Autodesk Inventor part; units mm, degrees
ref_plane "YZ Plane" through (0, 0, 0) normal (1, 0, 0) x (0, 1, 0)
ref_plane "XZ Plane" through (0, 0, 0) normal (0, 1, 0) x (-1, 0, 0)
ref_plane "XY Plane" through (0, 0, 0) normal (0, 0, 1) x (1, 0, 0)
sketch "草图1" plane through (0, 0, 0) normal (0, 0, 1) x (1, 0, 0)
  line L0 (-50, -50) -> (50, -50)
  line L1 (50, -50) -> (50, 50)
  line L2 (50, 50) -> (-50, 50)
  line L3 (-50, 50) -> (-50, -50)
  line L4 (-50, -50) -> (50, 50) construction
  line L5 (50, -50) -> (-50, 50) construction
  line L6 (-50, -50) -> (50, -50)
  line L7 (50, -50) -> (50, -65)
  line L8 (50, -65) -> (-50, -65)
  line L9 (-50, -65) -> (-50, -50)
  point P0 (0, 0)
  dimension "d0" = 100
  dimension "d1" = 100
  dimension "d2" = 15
extrude "拉伸1" add sketch "草图1" along normal blind 6
sketch "草图2" plane through (0, 0, 6) normal (0, 0, 1) x (1, 0, 0)
  line L0 (-25, -25) -> (25, -25)
  line L1 (25, -25) -> (25, 25)
  line L2 (25, 25) -> (-25, 25)
  line L3 (-25, 25) -> (-25, -25)
  line L4 (-25, -25) -> (25, 25) construction
  line L5 (25, -25) -> (-25, 25) construction
  point P0 (0, 0)
  dimension "d5" = 50
  dimension "d6" = 50
extrude "拉伸2" add sketch "草图2" along normal blind 6
sketch "草图3" plane through (0, 0, 12) normal (0, 0, 1) x (1, 0, 0)
  line L0 (-17.5, -17.5) -> (17.5, -17.5)
  line L1 (17.5, -17.5) -> (17.5, 17.5)
  line L2 (17.5, 17.5) -> (-17.5, 17.5)
  line L3 (-17.5, 17.5) -> (-17.5, -17.5)
  line L4 (-17.5, -17.5) -> (17.5, 17.5) construction
  line L5 (17.5, -17.5) -> (-17.5, 17.5) construction
  point P0 (0, 0)
  dimension "d9" = 35
  dimension "d10" = 35
extrude "拉伸3" cut sketch "草图3" against normal through all
sketch "草图4" plane through (0, 0, 12) normal (0, 0, 1) x (1, 0, 0)
  line L0 (-21, -21) -> (21, -21)
  line L1 (21, -21) -> (21, 21)
  line L2 (21, 21) -> (-21, 21)
  line L3 (-21, 21) -> (-21, -21)
  line L4 (-21, -21) -> (21, 21) construction
  line L5 (21, -21) -> (-21, 21) construction
  circle A0 centre (21, 21) radius 2.15
  circle A1 centre (-21, 21) radius 2.15
  circle A2 centre (-21, -21) radius 2.15
  circle A3 centre (21, -21) radius 2.15
  point P0 (0, 0)
  dimension "d13" = 42
  dimension "d14" = 42
  dimension "d15" = 4.3
  dimension "d16" = 4.3
  dimension "d17" = 4.3
  dimension "d18" = 4.3
extrude "拉伸4" cut sketch "草图4" against normal through all contours L3 A2 L0 | L0 A2 L3 | A3 L1 L0 | L0 L1 A3 | A1 L2 L3 | L3 L2 A1 | A0 L2 L1 | L1 L2 A0
sketch "草图5" plane through (0, 0, 0) normal (0, 0, -1) x (-1, 0, 0)
  line L0 (0, 0) -> (15, 0)
  line L1 (15, -17.5) -> (15, -57.5)
  line L2 (15, -57.5) -> (0, -57.5)
  line L3 (-17.5, -17.5) -> (17.5, -17.5)
  line L4 (15, -17.5) -> (0, -17.5)
  line L5 (-15, -17.5) -> (-15, -57.5)
  line L6 (-15, -57.5) -> (0, -57.5)
  line L7 (17.5, -17.5) -> (-17.5, -17.5)
  line L8 (0, -57.5) -> (10, -57.5)
  line L9 (10, -57.5) -> (10, -76.7389)
  line L10 (10, -76.7389) -> (0, -76.7389)
  line L11 (0, -76.7389) -> (0, -57.5)
  line L12 (-10, -57.5) -> (-10, -76.7389)
  line L13 (-10, -76.7389) -> (0, -76.7389)
  dimension "d21" = 15
  dimension "d22" = 40
  dimension "d23" = 10
extrude "拉伸5" cut sketch "草图5" against normal blind 3
sketch "草图6" plane through (0, 0, 0) normal (0, 0, -1) x (-1, 0, 0)
  point P0 (0, 0)
sketch "草图7" plane through (-50, -65, 6) normal (0, -1, 0) x (1, 0, 0)
  line L0 (100, -6) -> (0, -6)
  line L1 (0, -6) -> (0, 0)
  line L2 (100, -6) -> (0, -6)
  line L3 (0, -6) -> (0, 0)
  line L4 (0, 0) -> (100, 0)
  line L5 (100, 0) -> (100, -6)
  point P0 (50, -6)
extrude "拉伸6" add sketch "草图7" along normal blind 80
sketch "草图8" plane through (0, 0, 0) normal (0, 0, -1) x (-1, 0, 0)
  line L0 (10, -65) -> (-10, -65)
  line L1 (50, 50) -> (50, -145)
  line L2 (0, -65) -> (50, -65)
  line L3 (50, -65) -> (50, -145)
  line L4 (50, -145) -> (0, -145)
  line L5 (0, -145) -> (0, -65)
  line L6 (-50, 50) -> (-50, -145)
  line L7 (0, -65) -> (-50, -65)
  line L8 (-50, -145) -> (0, -145)
  point P0 (0, 0)
extrude "拉伸7" cut sketch "草图8" against normal blind 3
sketch "草图9" plane through (0, 0, 3) normal (0, 0, -1) x (-1, 0, 0)
  line L0 (-50, -145) -> (-50, -65)
  line L1 (-50, -65) -> (-47, -65)
  line L2 (-47, -65) -> (-47, -142)
  line L3 (-47, -155.7604) -> (-50, -155.7604)
  line L4 (-50, -145) -> (-50, -65)
  line L5 (50, 50) -> (50, -145)
  line L6 (50, -65) -> (47, -65)
  line L7 (47, -65) -> (47, -142)
  line L8 (47, -155.7604) -> (50, -155.7604)
  line L9 (50, -145) -> (50, -65)
  line L10 (-47, -142) -> (47, -142)
  line L11 (63.4475, -142) -> (63.4475, -145)
  line L12 (50, -145) -> (-50, -145)
  line L13 (-50, -145) -> (-50, -142)
  point P0 (0, 0)
  point P1 (50, -145)
  dimension "d30" = 3
  dimension "d31" = 3
  dimension "d32" = 3
extrude "拉伸8" add sketch "草图9" along normal blind 50
sketch "草图10" plane through (0, 0, -47) normal (0, 0, -1) x (-1, 0, 0)
  line L0 (50, -65) -> (47, -65)
  line L1 (50, -145) -> (50, -65)
  line L2 (-50, 50) -> (-50, -145)
  line L3 (-50, -145) -> (50, -145)
  line L4 (50, -145) -> (50, -65)
  line L5 (50, -65) -> (-50, -65)
  line L6 (-50, -65) -> (-50, -145)
  point P0 (0, 0)
extrude "拉伸9" add sketch "草图10" along normal blind 3
sketch "草图11" plane through (-50, 50, 0) normal (-1, 0, 0) x (0, 0, 1)
  line L0 (-42.728, -178.1257) -> (-27.728, -178.1257)
  line L1 (-27.728, -178.1257) -> (-27.728, -188.1257)
  line L2 (-27.728, -188.1257) -> (-42.728, -188.1257)
  line L3 (-42.728, -188.1257) -> (-42.728, -178.1257)
  point P0 (0, -50)
  dimension "d37" = 10
  dimension "d38" = 15
extrude "拉伸10" cut sketch "草图11" against normal blind 3
sketch "草图12" plane through (-50, -145, 6) normal (0, -1, 0) x (1, 0, 0)
  line L0 (0, -56) -> (100, -56)
  line L1 (100, -6) -> (100, -56)
  line L2 (100, -6) -> (97, -6)
  line L3 (100, -6) -> (100, -56)
  line L4 (0, -56) -> (100, -56)
  line L5 (0, -6) -> (0, -56)
  line L6 (3, -6) -> (0, -6)
  line L7 (3, -6) -> (3, -53)
  line L8 (3, -53) -> (97, -53)
  line L9 (97, -6) -> (97, -53)
  line L10 (100, -56) -> (0, -56)
  line L11 (0, -56) -> (0, -6)
  line L12 (0, -6) -> (100, -6)
  line L13 (100, -6) -> (100, -56)
  point P0 (50, -6)
sketch "草图13" plane through (0, 0, -50) normal (0, 0, -1) x (-1, 0, 0)
  line L0 (50, -145) -> (50, -65)
  line L1 (50, -65) -> (-50, -65)
  line L2 (-53.2797, -65) -> (-53.2797, -62)
  line L3 (-50, -62) -> (50, -62)
  line L4 (50, -62) -> (50, -65)
  line L5 (-50, 50) -> (-50, -65)
  line L6 (-50, -62) -> (-50, -65)
  line L7 (-50, 50) -> (-50, -65)
  line L8 (-50, 50) -> (-50, -145)
  line L9 (-50, -65) -> (-50, -145)
  line L10 (-50, 50) -> (-50, -65)
  line L11 (-50, 50) -> (-50, -145)
  line L12 (-50, -65) -> (-50, -145)
  point P0 (0, 0)
  dimension "d41" = 3
sketch "草图14" plane through (0, 0, 0) normal (0, 0, -1) x (-1, 0, 0)
  point P0 (0, 0)
extrude "拉伸11" add sketch "草图13" against normal blind 50
sketch "草图15" plane through (-50, -62, -50) normal (0, 1, 0) x (1, 0, 0)
  line L0 (50, -50) -> (35, -50)
  line L1 (35, -50) -> (35, -38)
  line L2 (35, -38) -> (50, -38)
  line L3 (50, -38) -> (50, -50)
  line L4 (50, -50) -> (65, -50)
  line L5 (65, -50) -> (65, -38)
  line L6 (65, -38) -> (50, -38)
  dimension "d44" = 15
  dimension "d45" = 12
extrude "拉伸12" cut sketch "草图15" against normal blind 10
sketch "草图16" plane through (-50, -145, 6) normal (0, -1, 0) x (1, 0, 0)
  line L0 (50, -6) -> (50, -31)
  line L1 (100, -56) -> (0, -56)
  circle A0 centre (50, -31) radius 3.15
  dimension "d48" = 25
  dimension "d49" = 6.3
extrude "拉伸13" cut sketch "草图16" against normal blind 10
sketch "草图17" plane through (0, 0, 12) normal (0, 0, 1) x (1, 0, 0)
  line L0 (17.5, 17.5) -> (-17.5, 17.5)
  line L1 (-17.5, -17.5) -> (17.5, -17.5)
  line L2 (17.5, -17.5) -> (17.5, 17.5)
  line L3 (17.5, 17.5) -> (-17.5, 17.5)
  line L4 (-17.5, 17.5) -> (-17.5, -17.5)
  line L5 (-17.5, -17.5) -> (17.5, 17.5) construction
  line L6 (17.5, -17.5) -> (-17.5, 17.5) construction
  line L7 (-12.5, -12.5) -> (12.5, -12.5)
  line L8 (12.5, -12.5) -> (12.5, 12.5)
  line L9 (12.5, 12.5) -> (-12.5, 12.5)
  line L10 (-12.5, 12.5) -> (-12.5, -12.5)
  line L11 (-12.5, -12.5) -> (12.5, 12.5) construction
  line L12 (12.5, -12.5) -> (-12.5, 12.5) construction
  point P0 (0, 0)
  dimension "d52" = 25
  dimension "d53" = 25
extrude "拉伸14" add sketch "草图17" against normal blind 12
sketch "草图18" plane through (0, 0, 0) normal (0, 0, -1) x (-1, 0, 0)
  line L0 (-15, -17.5) -> (15, -17.5)
  line L1 (-15, -17.5) -> (15, -17.5)
  line L2 (15, -17.5) -> (15, -12.5)
  line L3 (15, -12.5) -> (-15, -12.5)
  line L4 (-15, -12.5) -> (-15, -17.5)
  point P0 (0, 0)
  point P1 (15, -17.5)
  dimension "d56" = 5
extrude "拉伸15" cut sketch "草图18" against normal blind 3
sketch "草图19" plane through (-50, -62, -50) normal (0, 1, 0) x (1, 0, 0)
  line L0 (35, -50) -> (35, -38)
  line L1 (35, -38) -> (65, -38)
  line L2 (65, -38) -> (65, -50)
  line L3 (100, -50) -> (65, -50)
  line L4 (100, 0) -> (100, -50)
  line L5 (0, 0) -> (100, 0)
  line L6 (0, 0) -> (0, -50)
  line L7 (35, -50) -> (0, -50)
  line L8 (35, -50) -> (35, -38)
  line L9 (35, -38) -> (65, -38)
  line L10 (65, -38) -> (65, -50)
  line L11 (100, -50) -> (65, -50)
  line L12 (100, 0) -> (100, -50)
  line L13 (0, 0) -> (100, 0)
  line L14 (0, 0) -> (0, -50)
  line L15 (35, -50) -> (0, -50)
  line L16 (50, -50) -> (77.5, -50)
  line L17 (77.5, -50) -> (77.5, -20)
  line L18 (77.5, -20) -> (50, -20)
  line L19 (50, -20) -> (50, -50)
  line L20 (50, -50) -> (22.5, -50)
  line L21 (22.5, -50) -> (22.5, -20)
  line L22 (22.5, -20) -> (50, -20)
  dimension "d59" = 27.5
  dimension "d60" = 30
extrude "拉伸16" cut sketch "草图19" against normal blind 3 contours L7 L21 L22 L19 L1 L0 | L19 L18 L17 L3 L2 L1
sketch "草图20" plane through (-50, -145, 6) normal (0, -1, 0) x (1, 0, 0)
  circle A0 centre (50, -31) radius 3.15
  circle A1 centre (50, -31) radius 3.15
  line L0 (100, -56) -> (100, 0)
  line L1 (100, 0) -> (0, 0)
  line L2 (0, 0) -> (0, -56)
  line L3 (100, -56) -> (0, -56)
  circle A2 centre (50, -31) radius 3.15
  line L4 (100, -56) -> (0, -56)
  line L5 (0, -56) -> (0, 0)
  line L6 (0, 0) -> (100, 0)
  line L7 (100, 0) -> (100, -56)
  point P0 (50, -6)
extrude "拉伸17" add sketch "草图20" along normal blind 10
sketch "草图21" plane through (0, 0, 12) normal (0, 0, 1) x (1, 0, 0)
  line L0 (-17.5, -17.5) -> (17.5, -17.5)
  line L1 (17.5, -17.5) -> (17.5, 17.5)
  line L2 (17.5, 17.5) -> (-17.5, 17.5)
  line L3 (-17.5, 17.5) -> (-17.5, -17.5)
  line L4 (-17.5, -17.5) -> (17.5, 17.5) construction
  line L5 (17.5, -17.5) -> (-17.5, 17.5) construction
  point P0 (0, 0)
  dimension "d65" = 35
  dimension "d66" = 35
extrude "拉伸18" cut sketch "草图21" against normal blind 15
sketch "草图22" plane through (0, 0, 0) normal (0, 0, -1) x (-1, 0, 0)
  point P0 (0, 0)
properties part number "12"
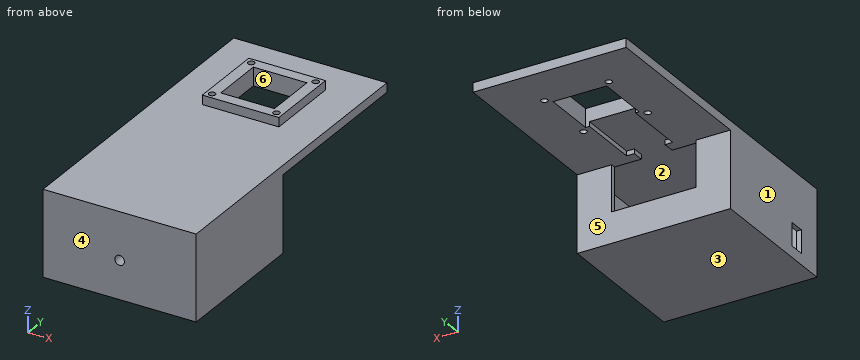
Build history of the part. All positions in model axes, mm. Face numbers are marked on the shaded views. A direction names the side the tool comes from. Round coordinates to 2 decimals unless told otherwise and drop trailing zeros. Loops run counter-clockwise (first coordinate to the right, second up) from the corner with the lowest first, then second, coordinate; pieces in that order, holes last. Notation, with made-up numbers: (19.25, 56) -> (65.25, 56) arc R23 cw to (65.25, 90) -> close; hole circle Ø8 at (61.25, 17.5). An arc over 180 degrees is marked (long way). Use CSV: the item, a comma, the result in double quotes. Start each with the question number.
Q1. Saw through at A-A on y = 21. Give the cut face in (x, z).
Q2. Saw through at C-C on z = -25. Give the cut face in (x, y).
Q3. Flat gauge pins, fed straight in: pin 1 Ø3.5 at (x, y) = (11.5, -63.5) entering from +Z; pin 2 Ø1.5 at (x, z) = (-48, -36) entering from +Y; pin 3 Ø2 at (x, y) = (-6.5, 24) entering from -Z; pin 4 Ø3.5 at (x, y) = (-21, 21) entering from +Z. Where does each tip first touch, or does it go through?
Q4. Saw through at B-B on x = 0. Give the cut face in (y, z), and give its area (3 significant figures).
Q5. Mould opens along Y. For the marked faces 3, 4, 5 and 6 say: +Y half, -Y half, draft (parallel to the pull), parting line (faces both ways), or undercut.
Q6. Saw through at D-D on x = -37.5. Give the cut face in (y, z).
Q7. Which spindle directions (+Z, -Z, +X, -X, +Y, -Y) get a long thin tool onto all of the face, cutting with end or side? Do the marked faces 1 and 2. Say none if no direction does.
Q8. Drill centre lines: L1, parallel to X at y = -21, z = 8; L2, parallel to X at y = -21, z = 5; L3, parallel to Y at x = -17, z = 0.5. Where is each one in solid material? Low to high.
Solutions:
1,outline,"(-50, 0) -> (-23.15, 0) -> (-23.15, 12) -> (-25, 12) -> (-25, 6) -> (-50, 6) -> close; (-18.85, 0) -> (18.85, 0) -> (18.85, 12) -> (-18.85, 12) -> close; (23.15, 0) -> (50, 0) -> (50, 6) -> (25, 6) -> (25, 12) -> (23.15, 12) -> close"
2,outline,"(-50, -155) -> (-3.15, -155) -> (-3.15, -142) -> (-47, -142) -> (-47, -65) -> (-27.5, -65) -> (-27.5, -62) -> (-50, -62) -> close; (3.15, -155) -> (50, -155) -> (50, -62) -> (27.5, -62) -> (27.5, -65) -> (47, -65) -> (47, -142) -> (3.15, -142) -> close"
3,pin 1,"stops at z = 6"
3,pin 2,"stops at y = -62"
3,pin 3,"stops at z = 0"
3,pin 4,"passes through"
4,outline,"(-155, -50) -> (-62, -50) -> (-62, -30) -> (-65, -30) -> (-65, -47) -> (-142, -47) -> (-142, -28.15) -> (-155, -28.15) -> close; (-155, -21.85) -> (-142, -21.85) -> (-142, 3) -> (-17.5, 3) -> (-17.5, 12) -> (-25, 12) -> (-25, 6) -> (-155, 6) -> close; (17.5, 0) -> (50, 0) -> (50, 6) -> (25, 6) -> (25, 12) -> (17.5, 12) -> close"
4,area,"1,600 mm^2"
5,face 3,"draft"
5,face 4,"-Y half"
5,face 5,"+Y half"
5,face 6,"undercut"
6,outline,"(-155, -50) -> (-62, -50) -> (-62, 0) -> (50, 0) -> (50, 6) -> (-155, 6) -> close; hole (-142, -47) -> (-65, -47) -> (-65, 3) -> (-142, 3) -> close"
7,face 1,"+Z, -Z, -X, +Y, -Y"
7,face 2,"none"
8,L1,"x = -25 to -23.15, -18.85 to 18.85, 23.15 to 25"
8,L2,"x = -50 to -23.15, -18.85 to 18.85, 23.15 to 50"
8,L3,"y = -155 to -142, -65 to -17.5, 17.5 to 50"
